from build123d import *

# Parameters (mm, degrees)
SKETCH_W      = 54
SKETCH_H      = 14
PAD_DEPTH     = 3
SKETCH001_R   = 4.5
SKETCH001_R_2 = 4
SKETCH001_R_3 = 5
PAD001_DEPTH  = 52
SKETCH002_R   = 4
SKETCH002_R_2 = 3.5
SKETCH002_R_3 = 3
PAD002_DEPTH  = 2
SKETCH003_R   = 5
SKETCH003_R_2 = 4.5
SKETCH003_R_3 = 4
PAD003_DEPTH  = 3
CHAMFER_SIZE  = 0.99


with BuildPart() as part:
    # Sketch → Pad (new body)
    with BuildSketch(Plane.XY):
        Rectangle(SKETCH_W, SKETCH_H)
    extrude(amount=PAD_DEPTH)

    # Sketch001 (on Face6 of Pad) → Pad001 (join)
    with BuildSketch(Plane.XY.offset(3)):
        Circle(SKETCH001_R)
        with Locations((17, 0)):
            Circle(SKETCH001_R_2)
        with Locations((-17, 0)):
            Circle(SKETCH001_R_3)
    extrude(amount=PAD001_DEPTH)

    # Sketch002 (on Face10 of Pad001) → Pad002 (join)
    with BuildSketch(Plane.XY.offset(55)):
        with Locations((-17, 0)):
            Circle(SKETCH002_R)
        Circle(SKETCH002_R_2)
        with Locations((17, 0)):
            Circle(SKETCH002_R_3)
    extrude(amount=PAD002_DEPTH)

    # Sketch003 (on Face16 of Pad002) → Pad003 (join)
    with BuildSketch(Plane.XY.offset(57)):
        with Locations((-17, 0)):
            Circle(SKETCH003_R)
        Circle(SKETCH003_R_2)
        with Locations((17, 0)):
            Circle(SKETCH003_R_3)
    extrude(amount=PAD003_DEPTH)

    # Chamfer
    chamfer_edges = [part.edges().sort_by_distance(p)[0] for p in [
        (-4.5, 0, 60),
        (13, 0, 60),
        (-22, 0, 60),
        (-21, 0, 57),
        (-3.5, 0, 57),
        (14, 0, 57),
        (-21, 0, 55),
        (-3.5, 0, 55),
        (14, 0, 55),
    ]]
    chamfer(chamfer_edges, length=CHAMFER_SIZE)


solid = part.part
Geometry check sheet. Reference: the model listing, model coordinates, mm. A direction names the side the tool comes from. Round coordinates to 2 decimals unless told otherwise and drop trailing zeros. Loops run counter-clockwise (first coordinate to the right, second up) from the corner with the lowest first, then second, coordinate; pieces in that order, holes last.
Item 1: Access from +Z, -Z, +X, -X, +Y, -Y to the whole of each face (thin tool, end or side, straight path). Record for faces 1 (the flat face through (0, -7, 1)), 2 (the cylindrical face through (-0.59, 4.46, 57.99)).
Item 2: Cross-section at B-B on z = 44. Record the boundary of the cut face in (x, y), then the cut area to 3 significant figures.
Item 3: Thickness scan on line 1 (X direction, y = -3.5, z = 41); line 2 (X direction, y = 1.5, z = 37); line 3 (Z direction, x = -25, y = 2.25). Record the ranges inside material, lowest first.
Item 4: Mould release check, pull along X, two halves, no side actions. Record for faces 3 (the flat face through (0, 5, 3)), 4 (the flat face through (17, 0, 60)), 5 (the flat face through (-27, 0, 1)): pulls with the +X half, pulls with the -X half, needs draft (parallel to the pull), parting line crosses it, or undercut.
Item 5: Gauge pin test, flat ends, axial feed: pin 1 (3 mm diameter, centred on y = -4, z = 29.5, fed in from +X); pin 2 (6.5 mm diameter, centred on x = 18.5, y = 0, fed in from -Z); pin 3 (1.5 mm diameter, centred on y = -2.5, z = 15, fed in from +X); pin 4 (2 mm diameter, centred on y = -2, z = 35, fed in from +X). Record the tip position at first contact, or that the pin passes through.
Answer sheet:
1. face 1: +Z, -Z, +X, -X, -Y
1. face 2: +Z
2. outline: circle Ø10 at (-17, 0); circle Ø9 at (0, 0); circle Ø8 at (17, 0)
2. area: 192 mm2
3. line 1: x = -20.57 to -13.43, -2.83 to 2.83, 15.06 to 18.94
3. line 2: x = -21.77 to -12.23, -4.24 to 4.24, 13.29 to 20.71
3. line 3: z = 0 to 3
4. face 3: undercut
4. face 4: needs draft
4. face 5: pulls with the -X half
5. pin 1: stops at x = 20.12
5. pin 2: stops at z = 0
5. pin 3: stops at x = 20.6
5. pin 4: stops at x = 20.87
